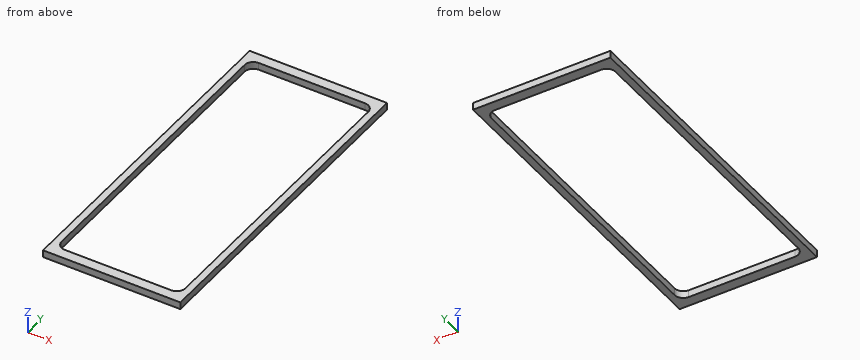
from build123d import *

# Parameters (mm, degrees)
SKETCH1_W           = 50.8
SKETCH1_H           = 121.92
BOSS_EXTRUDE1_DEPTH = 2.667
CUT_EXTRUDE1_DEPTH  = 67.093830945


with BuildPart() as part:
    # Sketch1 → Boss-Extrude1 (new body)
    with BuildSketch(Plane.XY):
        Rectangle(SKETCH1_W, SKETCH1_H)
    extrude(amount=BOSS_EXTRUDE1_DEPTH)

    # Sketch2 → Cut-Extrude1 (cut, through all)
    with BuildSketch(Plane.XY.offset(2.667)):
        with BuildLine():
            Line((19.685, -57.15), (-19.685, -57.15))
            ThreePointArc((-19.685, -57.15), (-21.93006403, -56.22006403), (-22.86, -53.975))
            Line((-22.86, -53.975), (-22.86, 53.975))
            ThreePointArc((-22.86, 53.975), (-21.93006403, 56.22006403), (-19.685, 57.15))
            Line((-19.685, 57.15), (19.685, 57.15))
            ThreePointArc((19.685, 57.15), (21.93006403, 56.22006403), (22.86, 53.975))
            Line((22.86, 53.975), (22.86, -53.975))
            ThreePointArc((22.86, -53.975), (21.93006403, -56.22006403), (19.685, -57.15))
        make_face()
    extrude(amount=-CUT_EXTRUDE1_DEPTH, mode=Mode.SUBTRACT)


solid = part.part
Check sheet for the modelled part. Datum: model origin and axes. Units: mm. Give positions to 0.01 mm unless a question says otherwise; leave off trailing zeros. Write each loop counter-clockwise with the first axis right and the second up, starting at its lowest first coordinate (ties: lowest second). Pieces come first, ordered by that corner, then holes. Notation, with made-up numbers: (76, 49.5) -> (120, 49.5) arc R8 ccw to (120, 61.5) -> close; hole circle Ø1 at (14, 64.5). An arc over 180 degrees is marked (long way). Write item = value, one per line.
Item 1: Sectioned sample at A-A on x = 7. Record the boundary of the cut face in (y, z), and give its area (3 significant figures).
Output:
outline = (-60.96, 0) -> (-57.15, 0) -> (-57.15, 2.67) -> (-60.96, 2.67) -> close; (57.15, 0) -> (60.96, 0) -> (60.96, 2.67) -> (57.15, 2.67) -> close
area = 20.3 mm^2
Item 2: Sectioned sample at B-B on y = -16.5. Record the boundary of the cut face in (x, z).
Output:
outline = (-25.4, 0) -> (-22.86, 0) -> (-22.86, 2.67) -> (-25.4, 2.67) -> close; (22.86, 0) -> (25.4, 0) -> (25.4, 2.67) -> (22.86, 2.67) -> close
Item 3: Scan lines: probe 1 along X at (y, z) = (46, 0.25); probe 2 along Y at (x, z) = (12.5, 0.8); probe 3 along Y at (x, z) = (22.5, 0.5). Record each from-to range of solid material in increasing order. Write a range as from..to.
Output:
probe_1 = -25.4..-22.86, 22.86..25.4
probe_2 = -60.96..-57.15, 57.15..60.96
probe_3 = -60.96..-55.44, 55.44..60.96
Item 4: Sectioned sample at C-C on z = 0.45. Record the boundary of the cut face in (x, y) (3 decimals).
Output:
outline = (-25.4, -60.96) -> (25.4, -60.96) -> (25.4, 60.96) -> (-25.4, 60.96) -> close; hole (-22.86, -53.975) arc R3.175 ccw to (-19.685, -57.15) -> (19.685, -57.15) arc R3.175 ccw to (22.86, -53.975) -> (22.86, 53.975) arc R3.175 ccw to (19.685, 57.15) -> (-19.685, 57.15) arc R3.175 ccw to (-22.86, 53.975) -> close
